Can you work these out from the drawing? Everything is in mm from the part's minimum corner. A direction names the side the tool comes from. Give positions to 0.01 mm unless a question says otherwise; leave off trailing zeros. Write each loop counter-clockwise with the first axis right and the second up, starting at its lowest first coordinate (ties: lowest second). Pieces come first, ordered by that corner, then holes. Notation, with made-up numbers: M 30.5,-35 L 48.5,-35 A12 ccw 48.5,-31 Z; hole C -22.5,84 d7. An arc over 180 degrees is marked long. One line per item, written item: value.
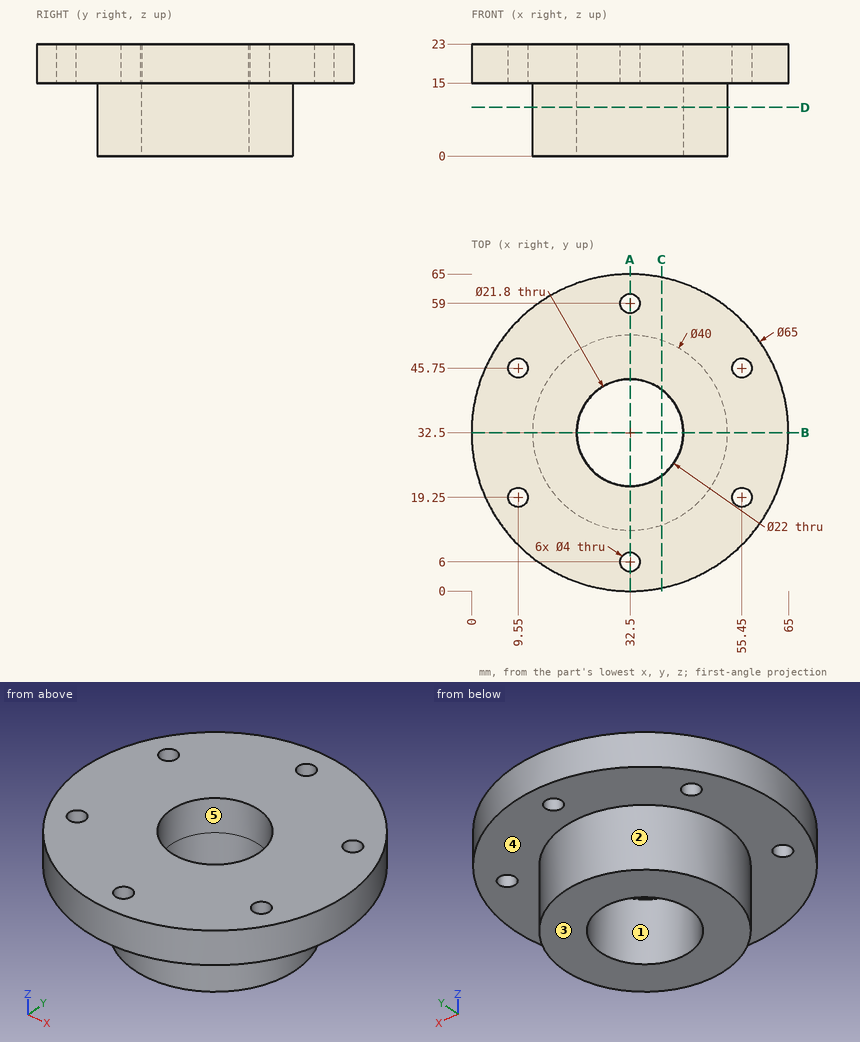
1) If we section it at D-D, the plane z = 10: Write out the boundary of the cut face in (x, y).
Outcome:
outline: C 32.5,32.5 d40; hole C 32.5,32.5 d22
2) Please list where these lines run through material, in increasing order: L1, parallel to X at y = 44, z = 18 (1 decimal); L2, parallel to Z at x = 48, y = 4.5; L3, parallel to Y at x = 32.5, z = 4.25. Write a range as from..to.
Outcome:
L1: x = 2.1..8.6, 10.5..54.5, 56.4..62.9
L2: z = 15..23
L3: y = 12.5..21.5, 43.5..52.5
3) We'd pull the mould along Y, two halves only. Please class the marked faces 1, 2 and 3: pulls with the +Y half, pulls with the -Y half, needs draft (parallel to the pull), parting line crosses it, or undercut.
Outcome:
face 1: undercut
face 2: parting line crosses it
face 3: needs draft
4) If we section it at A-A, the plane x = 32.5: Write out the boundary of the cut face in (y, z).
Outcome:
outline: M 0,15 L 4,15 L 4,23 L 0,23 Z; M 8,15 L 12.5,15 L 12.5,0 L 21.5,0 L 21.5,15 L 21.6,15 L 21.6,23 L 8,23 Z; M 43.4,15 L 43.5,15 L 43.5,0 L 52.5,0 L 52.5,15 L 57,15 L 57,23 L 43.4,23 Z; M 61,15 L 65,15 L 65,23 L 61,23 Z
5) If we section it at B-B, the plane y = 32.5: Write out the boundary of the cut face in (x, z).
Outcome:
outline: M 0,15 L 12.5,15 L 12.5,0 L 21.5,0 L 21.5,15 L 21.6,15 L 21.6,23 L 0,23 Z; M 43.4,15 L 43.5,15 L 43.5,0 L 52.5,0 L 52.5,15 L 65,15 L 65,23 L 43.4,23 Z
6) On a 3-axis mill with a long thin cutter (end or side, diameter ignored), from which of +Z, -Z, +X, -X, +Y, -Y can I reach the whole of each face in a straight line? I mean the marked faces 4 and 5. Say none if no direction works.
Outcome:
face 4: -Z
face 5: +Z, -Z
7) If we section it at C-C, the plane x = 39: Write out the boundary of the cut face in (y, z), then the cut area to 3 significant figures.
Outcome:
outline: M 0.66,15 L 13.59,15 L 13.59,0 L 23.63,0 L 23.63,15 L 23.75,15 L 23.75,23 L 0.66,23 Z; M 41.25,15 L 41.37,15 L 41.37,0 L 51.41,0 L 51.41,15 L 64.34,15 L 64.34,23 L 41.25,23 Z
area: 671 mm^2
8) I'm going to push flat-ended pins straight in: pin 1 (12 mm diameter, centred on x = 56, z = 6, fed in from +Y); pin 2 (2 mm diameter, centred on x = 37, z = 20.5, fed in from -Y); pin 3 (4 mm diameter, centred on x = 27, z = 19, fed in from +Y); pin 4 (25 mm diameter, centred on x = 32.5, y = 32.5, fed in from +Z). Where does each tip first touch, or does it pass through?
Outcome:
pin 1: stops at y = 42.18
pin 2: stops at y = 0.19
pin 3: stops at y = 64.81
pin 4: stops at z = 23
